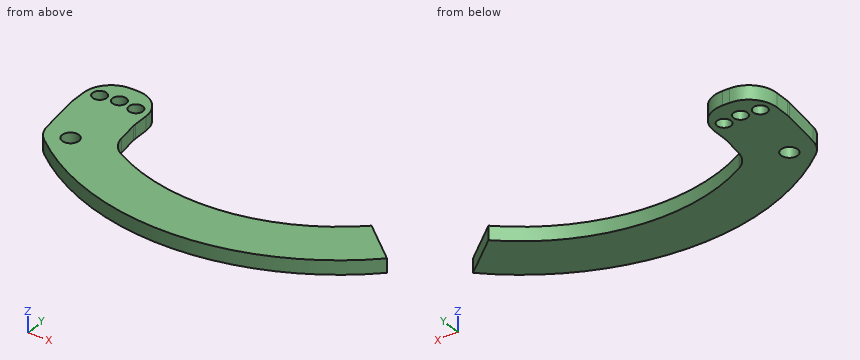
from build123d import *

# Parameters (mm, degrees)
ESQUISSE1_R        = 6
ESQUISSE1_R_2      = 5
BOSS_EXTRU_1_DEPTH = 5
CONG_1_R           = 20


with BuildPart() as part:
    # Esquisse1 → Boss.-Extru.1 (new body, symmetric)
    with BuildSketch(Plane.XY):
        with BuildLine():
            Line((200.083196535, -26.00073282), (228.193277133, -50.436453083))
            ThreePointArc((228.193277133, -50.436453083), (105.798406768, -100.555368837), (-17.5, -52.702334489))
            Line((-17.5, -52.702334489), (-22.5, -14.5))
            Line((-22.5, -14.5), (-22.5, 17.5))
            Line((-22.5, 17.5), (22.5, 17.5))
            Line((22.5, 17.5), (22.5, -14.5))
            Line((22.5, -14.5), (25.81470592, -39.825900861))
            ThreePointArc((25.81470592, -39.825900861), (115.339933121, -63.052032289), (200.083196535, -26.00073282))
        make_face()
        with Locations((0, -47.5)):
            Circle(ESQUISSE1_R, mode=Mode.SUBTRACT)
        with Locations((-12.940952255, 0.796291314)):
            Circle(ESQUISSE1_R_2, mode=Mode.SUBTRACT)
        with Locations((0, 2.5)):
            Circle(ESQUISSE1_R_2, mode=Mode.SUBTRACT)
        with Locations((12.940952255, 0.796291314)):
            Circle(ESQUISSE1_R_2, mode=Mode.SUBTRACT)
    extrude(amount=BOSS_EXTRU_1_DEPTH, both=True)

    # Congé1
    cong_1_edges = [part.edges().sort_by_distance(p)[0] for p in [
        (-17.5, -52.702334489, 0),
        (-22.5, -14.5, 0),
        (-22.5, 17.5, 0),
        (22.5, 17.5, 0),
        (22.5, -14.5, 0),
        (25.81470592, -39.825900861, 0),
    ]]
    fillet(cong_1_edges, radius=CONG_1_R)


solid = part.part
Check sheet for the modelled part. Datum: model origin and axes. Units: mm. Round coordinates to 2 decimals unless told otherwise and drop trailing zeros. Loops run counter-clockwise (first coordinate to the right, second up) from the corner with the lowest first, then second, coordinate; pieces in that order, holes last.
1. Gauge pin test, flat ends, axial feed: pin 1 Ø5 at (y, z) = (-34.5, 2.5) entering from -X; pin 2 Ø5 at (y, z) = (-6.5, -2) entering from +X; pin 3 Ø5 at (y, z) = (-68.5, -2.5) entering from +X; pin 4 Ø6 at (x, y) = (-12.94, 0.8) entering from +Z. Record the tip position at first contact, or that the pin passes through.
2. Scan lines: probe 1 along Y at (x, z) = (0, 2.5); probe 2 along X at (y, z) = (-51.5, -2.75); probe 3 along X at (y, z) = (-45, 4). Record each from-to range of solid material in increasing order.
3. Sectioned sample at A-A on y = -61. Record the boundary of the cut face in (x, z).
4. Sectioned sample at D-D on x = 173.5. Record the boundary of the cut face in (y, z).
5. Sectioned sample at C-C on x = 0. Record the boundary of the cut face in (y, z), and give its area (3 significant figures).
6. Sectioned sample at B-B on z = -3. Record the boundary of the cut face in (x, y).
Recorded:
1. pin 1: stops at x = -20.21
1. pin 2: stops at x = 22.5
1. pin 3: stops at x = 209.73
1. pin 4: passes through
2. probe 1: y = -67.04 to -53.5, -41.5 to -2.5, 7.5 to 17.5
2. probe 2: x = -16.61 to -4.47, 4.47 to 47.14, 161.16 to 227.08
2. probe 3: x = -18.51 to -5.45, 5.45 to 34.22, 174.09 to 221.94
3. outline: (-7.93, -5) - (77.7, -5) - (77.7, 5) - (-7.93, 5) - close; (130.6, -5) - (216.23, -5) - (216.23, 5) - (130.6, 5) - close
4. outline: (-86.54, -5) - (-45.33, -5) - (-45.33, 5) - (-86.54, 5) - close
5. outline: (-67.04, -5) - (-53.5, -5) - (-53.5, 5) - (-67.04, 5) - close; (-41.5, -5) - (-2.5, -5) - (-2.5, 5) - (-41.5, 5) - close; (7.5, -5) - (17.5, -5) - (17.5, 5) - (7.5, 5) - close
5. area: 625 mm2
6. outline: (-22.5, -13.2) arc R20 ccw to (-22.33, -15.79) - (-18.47, -45.32) arc R20 ccw to (-11.6, -57.95) arc R178.54 ccw to (228.19, -50.44) - (200.08, -26) arc R141.47 cw to (34.57, -45.2) arc R20 cw to (24.58, -30.38) - (22.67, -15.79) arc R20 cw to (22.5, -13.2) - (22.5, -2.5) arc R20 ccw to (2.5, 17.5) - (-2.5, 17.5) arc R20 ccw to (-22.5, -2.5) - close; hole circle Ø10 at (-12.94, 0.8); hole circle Ø12 at (0, -47.5); hole circle Ø10 at (0, 2.5); hole circle Ø10 at (12.94, 0.8)
